Source: three-view drawing plus pictorial views. Frame: mm from the lowest corner of the part. A direction names the side the tool comes from. Coordinates: 2 decimals unless noted, no trailing zeros. Loops run counter-clockwise (first coordinate to the right, second up) from the corner with the lowest first, then second, coordinate; pieces in that order, holes last. Notation, with made-up numbers: M 51,-33 L 81,-33 A16 ccw 81,-15 Z; hole C 79.25,24 d8. An arc over 180 degrees is marked long. Use a Markdown table: item, result. Add a question column.
1. Set-up query: the marked faces 4, 5 and 6. Return all of +Z, -Z, +X, -X, +Y, -Y with unobstructed straight access to the full face (end or side cutting, diameter ignored); none if empty.
2. Line query: L1, parallel to Z at x = 59.69, y = 2.05; L2, parallel to X at y = 20, z = 14; L3, parallel to X at y = 3.2, z = 31.75. Output: solid intervals per line, ascending. Write a range as [from, to].
3. Section C-C on y = 20.32. Output: boundary loops of the cut face in (x, z).
4. Draft query along Y for the marked faces 1, 2 and 3. Return one class per face: +Y half, -Y half, draft (parallel to the pull), parting line (faces both ways), or undercut.
5. Section A-A on x = 59.69. Output: boundary loops of the cut face in (y, z).
6. Section B-B on z = 15.5. Output: boundary loops of the cut face in (x, y).
7. Section D-D on z = 6.35. Output: boundary loops of the cut face in (x, y).
8. Pin query (flat end, axial travel): pin 1 (5.5 mm diameter, centred on y = 15.5, z = 9.5, fed in from -X); pin 2 (21 mm diameter, centred on y = 20.5, z = 27.5, fed in from +X); pin 3 (10 mm diameter, centred on x = 11, y = 14, fed in from -Z); pin 4 (4.5 mm diameter, centred on x = 4, z = 21, fed in from +Y). Return the tip coordinate at first contact, or that it passes through.
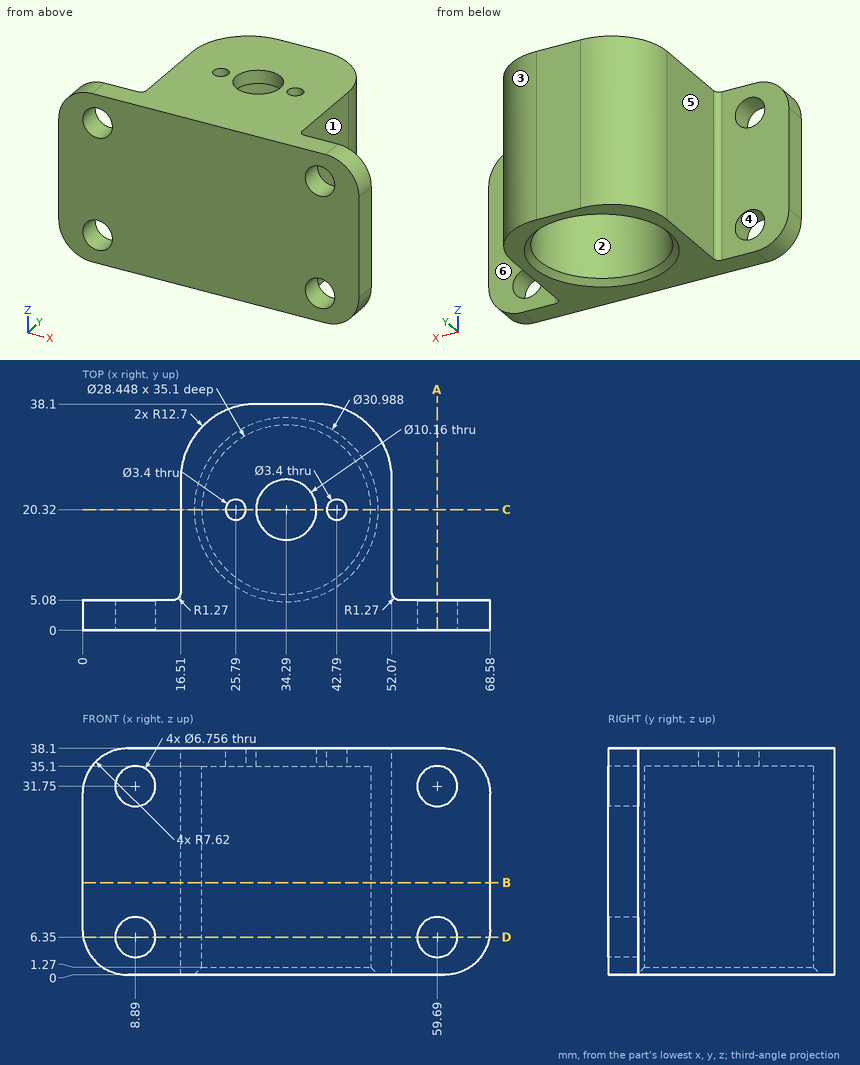
Answers below:
| question | item | result |
|---|---|---|
| 1 | face 4 | +Y, -Y |
| 1 | face 5 | +Z, -Z, -X, +Y |
| 1 | face 6 | +Z, -Z, +X, +Y |
| 2 | L1 | z = [0, 2.97], [9.73, 28.37], [35.13, 38.1] |
| 2 | L2 | x = [16.51, 20.07], [48.51, 52.07] |
| 2 | L3 | x = [0.11, 5.51], [12.27, 56.31], [63.07, 68.47] |
| 3 | outline | M 16.51,0 L 18.8,0 L 20.07,1.27 L 20.07,35.1 L 24.09,35.1 L 24.09,38.1 L 16.51,38.1 Z; M 27.49,35.1 L 29.21,35.1 L 29.21,38.1 L 27.49,38.1 Z; M 39.37,35.1 L 41.09,35.1 L 41.09,38.1 L 39.37,38.1 Z; M 44.49,35.1 L 48.51,35.1 L 48.51,1.27 L 49.78,0 L 52.07,0 L 52.07,38.1 L 44.49,38.1 Z |
| 4 | face 1 | draft |
| 4 | face 2 | undercut |
| 4 | face 3 | +Y half |
| 5 | outline | M 0,0 L 5.08,0 L 5.08,2.97 L 0,2.97 Z; M 0,9.73 L 5.08,9.73 L 5.08,28.37 L 0,28.37 Z; M 0,35.13 L 5.08,35.13 L 5.08,38.1 L 0,38.1 Z |
| 6 | outline | M 0,0 L 68.58,0 L 68.58,5.08 L 53.34,5.08 A1.27 cw 52.07,6.35 L 52.07,25.4 A12.7 ccw 39.37,38.1 L 29.21,38.1 A12.7 ccw 16.51,25.4 L 16.51,6.35 A1.27 cw 15.24,5.08 L 0,5.08 Z; hole C 34.29,20.32 d28.45 |
| 7 | outline | M 0.11,0 L 5.51,0 L 5.51,5.08 L 0.11,5.08 Z; M 12.27,0 L 56.31,0 L 56.31,5.08 L 53.34,5.08 A1.27 cw 52.07,6.35 L 52.07,25.4 A12.7 ccw 39.37,38.1 L 29.21,38.1 A12.7 ccw 16.51,25.4 L 16.51,6.35 A1.27 cw 15.24,5.08 L 12.27,5.08 Z; M 63.07,0 L 68.47,0 L 68.47,5.08 L 63.07,5.08 Z; hole C 34.29,20.32 d28.45 |
| 8 | pin 1 | stops at x = 16.51 |
| 8 | pin 2 | stops at x = 52.07 |
| 8 | pin 3 | passes through |
| 8 | pin 4 | stops at y = 5.08 |
